from build123d import *

# Parameters (mm, degrees)
BOSS_EXTRUDE1_DEPTH = 15.28
SKETCH2_R           = 4.05
BOSS_EXTRUDE2_DEPTH = 9.72
CHAMFER1_SIZE       = 9.72
CHAMFER1_SIZE_2     = 0.62
CHAMFER2_SIZE       = 9.72
CHAMFER2_SIZE_2     = 0.62
SKETCH4_W           = 9.08
SKETCH4_H           = 11.11
CUT_EXTRUDE1_DEPTH  = 30
SKETCH6_W           = 1.5
SKETCH6_H           = 3
SKETCH6_W_2         = 1.57
SKETCH6_W_3         = 1.38
SKETCH6_H_2         = 1.2
BOSS_EXTRUDE3_DEPTH = 25.04233017
SKETCH7_W           = 1.5
SKETCH7_H           = 3
CUT_EXTRUDE2_DEPTH  = 19.72
SKETCH8_R           = 3
CUT_EXTRUDE3_DEPTH  = 11.19
SKETCH9_W           = 11.6
SKETCH9_H           = 4.67
CUT_EXTRUDE4_DEPTH  = 32


with BuildPart() as part:
    # Sketch1 → Boss-Extrude1 (new body)
    with BuildSketch(Plane(origin=(0, 0, 0), x_dir=(1, 0, 0), z_dir=(0, 1, 0))):
        Polygon((-3.25, 5.8), (-15, 5.8), (-15, -5.8), (15, -5.8), (15, 5.8), (3.25, 5.8), align=None)
    extrude(amount=BOSS_EXTRUDE1_DEPTH)

    # Sketch2 → Boss-Extrude2 (add)
    with BuildSketch(Plane(origin=(0, 15.28, 0), x_dir=(1, 0, 0), z_dir=(0, 1, 0))):
        with Locations(Location((-5.98, 0, 0), (0, 0, 270))):
            Circle(SKETCH2_R)
        with Locations(Location((6.97, 0, 0), (0, 0, 270))):
            Circle(SKETCH2_R)
    extrude(amount=BOSS_EXTRUDE2_DEPTH)

    # Chamfer1
    # the kernel refuses this chamfer: 9.72, 0.62 mm, written as the material it takes off along each edge
    with BuildSketch(Plane(origin=(-5.98, 25, 0), x_dir=(0, 0, 1), z_dir=(-1, 0, 0))) as chamfer1_piece_1_section:
        Polygon((4.05, -CHAMFER1_SIZE), (4.05 - CHAMFER1_SIZE_2, 0), (4.05, 0), align=None)
    chamfer1_piece_1 = revolve(axis=Axis((-5.98, 25, 0), (0, 1, 0)), mode=Mode.PRIVATE)
    chamfer1_piece_1 = split(chamfer1_piece_1, bisect_by=Plane(origin=(-5.98, 15.28, -3.777775081), z_dir=(0, 1, 0)), keep=Keep.TOP, mode=Mode.PRIVATE)
    add(chamfer1_piece_1, mode=Mode.SUBTRACT)

    # Chamfer2
    # the kernel refuses this chamfer: 9.72, 0.62 mm, written as the material it takes off along each edge
    with BuildSketch(Plane(origin=(6.97, 25, 0), x_dir=(0, 0, 1), z_dir=(-1, 0, 0))) as chamfer2_piece_1_section:
        Polygon((4.05, -CHAMFER2_SIZE), (4.05 - CHAMFER2_SIZE_2, 0), (4.05, 0), align=None)
    chamfer2_piece_1 = revolve(axis=Axis((6.97, 25, 0), (0, 1, 0)), mode=Mode.PRIVATE)
    chamfer2_piece_1 = split(chamfer2_piece_1, bisect_by=Plane(origin=(6.97, 15.28, -3.777775081), z_dir=(0, 1, 0)), keep=Keep.TOP, mode=Mode.PRIVATE)
    add(chamfer2_piece_1, mode=Mode.SUBTRACT)

    # Sketch4 → Cut-Extrude1 (cut)
    with BuildSketch(Plane(origin=(15, 0, 0), x_dir=(0, 0, -1), z_dir=(1, 0, 0))):
        with Locations((0, 8.255)):
            Rectangle(SKETCH4_W, SKETCH4_H)
    extrude(amount=-CUT_EXTRUDE1_DEPTH, mode=Mode.SUBTRACT)

    # Sketch6 → Boss-Extrude3 (add)
    with BuildSketch(Plane.ZY.offset(15)):
        with Locations((0, 12.31)):
            Rectangle(SKETCH6_W, SKETCH6_H)
        with Locations((-3.755, 12.31)):
            Rectangle(SKETCH6_W_2, SKETCH6_H)
        with Locations((-2.66, 3.3)):
            Rectangle(SKETCH6_W_3, SKETCH6_H_2)
        with Locations((2.66, 3.3)):
            Rectangle(SKETCH6_W_3, SKETCH6_H_2)
        with Locations((3.755, 12.31)):
            Rectangle(SKETCH6_W_2, SKETCH6_H)
    extrude(amount=-BOSS_EXTRUDE3_DEPTH)

    # Sketch7 → Cut-Extrude2 (cut)
    with BuildSketch(Plane(origin=(10.04233017, 0, 0), x_dir=(0, 0, -1), z_dir=(1, 0, 0))):
        with Locations((0, 12.31)):
            Rectangle(SKETCH7_W, SKETCH7_H)
    extrude(amount=-CUT_EXTRUDE2_DEPTH, mode=Mode.SUBTRACT)

    # Sketch8 → Cut-Extrude3 (cut)
    with BuildSketch(Plane(origin=(0, 25, 0), x_dir=(1, 0, 0), z_dir=(0, 1, 0))):
        with Locations(Location((6.97, 0, 0), (0, 0, 270))):
            Circle(SKETCH8_R)
        with Locations(Location((-5.98, 0, 0), (0, 0, 270))):
            Circle(SKETCH8_R)
    extrude(amount=-CUT_EXTRUDE3_DEPTH, mode=Mode.SUBTRACT)

    # Sketch9 → Cut-Extrude4 (cut)
    with BuildSketch(Plane.ZY.offset(15)):
        with Locations((0, 22.665)):
            Rectangle(SKETCH9_W, SKETCH9_H)
    extrude(amount=-CUT_EXTRUDE4_DEPTH, mode=Mode.SUBTRACT)


solid = part.part
Design review of the part built by this model. Coordinates are the model's own, in mm. A direction names the side the tool comes from. Coordinates: 2 decimals unless noted, no trailing zeros. Order: outer loops, then holes, each group sorted by start corner. A loop starts at its lowest first (then second) coordinate and runs counter-clockwise, first axis right, second up.
Item 1: The part is to be moulded in two halves that separate along X. For faces 1 (the flat face through (0, 7, -4.54)), 2 (the flat face through (10.042, 12, 4)), 3 (the conical face through (-9.774, 17.84, -0.843)), say which applies: pulls with the +X half, pulls with the -X half, needs draft (parallel to the pull), parting line crosses it, or undercut.
Item 2: For line 1 (Z direction, x = 3, y = 2.75); line 2 (Z direction, x = -3, y = 11.5); line 3 (Z direction, x = 3.25, y = 9), list the stretches that pass through material, from the lowest coordinate up.
Item 3: For pin 1 Ø6 at (x, z) = (-1, -1.5) entering from +Y; pin 2 Ø0.5 at (y, z) = (12.5, 3.5) entering from +X, all flat-tipped, find the tip position at first contact; note any pin that passes through.
Item 4: Take a section at C-C, the plane x = 12. Write out the cut boundary in (y, z).
Item 5: Take a section at B-B, the plane z = 0. Write out the cut boundary in (x, y).
Item 6: Take a section at A-A, the plane y = 10.25. Write out the cut boundary in (x, z).
Item 7: For faces 4 (the flat face through (15, 2, 0)), 5 (the flat face through (-3, 3.9, 3)), 6 (the flat face through (1, 13.81, 0)), 7 (the cylindrical face through (-3.006, 17.116, -0.391)), list the 3-axis set-ups (+Z, -Z, +X, -X, +Y, -Y) from which the entire face can be reached by the end or side of a thin tool; tool diameter is ignored.
The answers:
1. face 1: needs draft
1. face 2: pulls with the +X half
1. face 3: undercut
2. line 1: z = -5.8 to -4.54, -3.35 to -1.97, 1.97 to 3.35, 4.54 to 5.8
2. line 2: z = -5.8 to -2.97, 2.97 to 5.8
2. line 3: z = -5.8 to -4.54, 4.54 to 5.8
3. pin 1: stops at y = 20.33
3. pin 2: stops at x = 10.04
4. outline: (0, -5.8) - (15.28, -5.8) - (15.28, 5.8) - (0, 5.8) - close; hole (2.7, -4.54) - (13.81, -4.54) - (13.81, 4.54) - (2.7, 4.54) - close
5. outline: (-15, 0) - (15, 0) - (15, 2.7) - (-15, 2.7) - close; (-15, 10.81) - (-9.68, 10.81) - (-9.68, 13.81) - (-8.98, 13.81) - (-8.98, 20.33) - (-9.71, 20.33) - (-10.03, 15.28) - (-15, 15.28) - close; (-2.98, 13.81) - (3.97, 13.81) - (3.97, 20.33) - (3.24, 20.33) - (2.92, 15.28) - (-1.93, 15.28) - (-2.25, 20.33) - (-2.98, 20.33) - close; (9.97, 13.81) - (15, 13.81) - (15, 15.28) - (11.02, 15.28) - (10.7, 20.33) - (9.97, 20.33) - close
6. outline: (-15, -5.8) - (15, -5.8) - (15, -4.54) - (-15, -4.54) - close; (-15, 4.54) - (15, 4.54) - (15, 5.8) - (-15, 5.8) - close
7. face 4: +Z, -Z, +X, +Y, -Y
7. face 5: +X, -X
7. face 6: +X
7. face 7: +Y
